Autodesk Fusion 360 part; units mm, degrees
sketch "Sketch1" plane through (0, 0, 0) normal (0, 1, 0) x (1, 0, 0)
  line L0 (-10, -10) -> (10, -10)
  line L1 (10, -10) -> (10, 10)
  line L2 (10, 10) -> (-10, 10)
  line L3 (-10, 10) -> (-10, -10)
  line L4 (0, 15) -> (15, 15)
  line L5 (15, -15) -> (-15, -15)
  line L6 (0, 15) -> (-15, 15)
  line L7 (0, -15) -> (15, -15)
  line L8 (0, -15) -> (-15, -15)
  line L9 (-15, 15) -> (15, 15)
  line L10 (-40, -12) -> (-18, -12)
  line L11 (-40, 12) -> (-18, 12)
  line L12 (40, 12) -> (18, 12)
  line L13 (40, -12) -> (18, -12)
  arc A0 (-40, 12) -> (-40, -12) centre (-40, 0) ccw
  line L14 (15, 15) -> (15, 15)
  line L15 (15, -15) -> (15, -15)
  arc A1 (40, -12) -> (40, 12) centre (40, 0) ccw
  line L16 (-15, -15) -> (-15, -15)
  line L17 (-15, 15) -> (-15, 15)
  circle A2 centre (-40, 0) radius 5
  circle A3 centre (40, 0) radius 5
  arc A4 (-18, 12) -> (-15, 15) centre (-18, 15) ccw
  arc A5 (15, 15) -> (18, 12) centre (18, 15) ccw
  arc A6 (18, -12) -> (15, -15) centre (18, -15) ccw
  arc A7 (-15, -15) -> (-18, -12) centre (-18, -15) ccw
  line L18 (-15, -15) -> (-15, 15)
  line L19 (15, 15) -> (15, -15)
  line L20 (52, 0) -> (52, 70) construction
  line L21 (-52, 0) -> (-52, 70) construction
  line L22 (0, 70) -> (-24.5, 70)
  line L23 (0, 70) -> (24.5, 70)
  line L24 (-15, 15) -> (-24.5, 70)
  line L25 (15, 15) -> (24.5, 70)
  dimension "d2" = 15
  dimension "d4" = 30
  dimension "d12" = 3
  dimension "d13" = 3
  dimension "d14" = 3
  dimension "d15" = 3
  dimension "d17" = 70
  dimension "d19" = 70
  dimension "d20" = 24.5
  dimension "d21" = 24.5
extrude "Extrude1" add sketch "Sketch1" along normal blind 15 and the other way blind 15 contours L4 L5 L6 L7 L8 L9 L18 L19
extrude "Extrude3" add sketch "Sketch1" along normal blind 5 contours L10 L11 A0 A4 A7 L18
extrude "Extrude4" add sketch "Sketch1" along normal blind 0 and the other way blind 5 contours L10 L11 A0 A4 A7 L18
extrude "Extrude5" add sketch "Sketch1" along normal blind 5 and the other way blind 5 contours L12 L13 A1 A5 A6 L19
extrude "Extrude6" add sketch "Sketch1" along normal blind 15 and the other way blind 7.5 contours L4 L6 L9 L22 L23 L24 L25
sketch "Sketch2" plane through (0, 0, 0) normal (1, 0, 0) x (0, 1, 0)
  line L0 (0, -15) -> (-7.5, -15)
  line L1 (-7.5, -15) -> (-7.5, -70)
  line L2 (-7.5, -70) -> (-30, -70)
  line L3 (-7.5, -15) -> (-30, -70)
  dimension "d44" = 7.5
  dimension "d45" = 22.5
extrude "Extrude7" add sketch "Sketch2" along normal blind 7.5 and the other way blind 7.5
sketch "Sketch3" plane through (0, 0, -70) normal (0, 0, -1) x (1, 0, 0)
  line L0 (-24.5, 7.5) -> (-24.5, -15)
  line L1 (-24.5, -15) -> (24.5, -15)
  line L2 (24.5, -15) -> (24.5, 7.5)
  line L3 (24.5, 7.5) -> (7.5, 7.5)
  line L4 (7.5, 7.5) -> (7.5, 30)
  line L5 (7.5, 30) -> (-7.5, 30)
  line L6 (-7.5, 30) -> (-7.5, 7.5)
  line L7 (-7.5, 7.5) -> (-24.5, 7.5)
  line L8 (0, -15) -> (45, -15)
  line L9 (45, -15) -> (-45, -15)
  line L10 (-45, 30) -> (45, 30)
  arc A0 (-45, -2.5) -> (-45, 17.5) centre (-45, 7.5) ccw
  arc A1 (-45, 17.5) -> (-45, -2.5) centre (-45, 7.5) ccw
  arc A2 (45, -2.5) -> (45, 17.5) centre (45, 7.5) ccw
  arc A3 (45, 17.5) -> (45, -2.5) centre (45, 7.5) ccw
  arc A4 (45, -15) -> (45, 30) centre (45, 7.5) ccw
  arc A5 (-45, 30) -> (-45, -15) centre (-45, 7.5) ccw
  line L11 (-24.5, -15) -> (24.5, -15)
  dimension "d51" = 22.5
  dimension "d52" = 20
  dimension "d53" = 20
extrude "Extrude8" add sketch "Sketch3" along normal blind 15
extrude "Extrude2" [suppressed]
The model under review builds one solid part; all positions refer to its coordinate system, in mm. A direction names the side the tool comes from. Round coordinates to 2 decimals unless told otherwise and drop trailing zeros. Order: outer loops, then holes, each group sorted by start corner. A loop starts at its lowest first (then second) coordinate and runs counter-clockwise, first axis right, second up. Notation, with made-up numbers: M 6.5,30.25 L 48.5,30.25 A16 ccw 48.5,49.25 Z; hole C -14,44.25 d5. An arc over 180 degrees is marked long. Use a Markdown table: item, result.
1) Consider section D-D (x = 42). Write out the cut boundary in (y, z).
Report:
| item | result |
|---|---|
| outline | M -30,-85 L -17.04,-85 L -17.04,-70 L -30,-70 Z; M -5,-11.83 L 5,-11.83 L 5,-4.58 L -5,-4.58 Z; M -5,4.58 L 5,4.58 L 5,11.83 L -5,11.83 Z; M 2.04,-85 L 15,-85 L 15,-70 L 2.04,-70 Z |
2) Consider section A-A (x = 5). Write out the cut boundary in (y, z), then the cut area to 3 significant figures.
Report:
| item | result |
|---|---|
| outline | M -30,-85 L 15,-85 L 15,-10 L -15,-10 L -15,-15 L -7.5,-15 L -30,-70 Z; M -15,10 L 15,10 L 15,15 L -15,15 Z |
| area | 2,830 mm^2 |
3) Wall thickness on line 1 along X through (y, z) = (0.5, 0); line 2 along X through (y, z) = (-7.5, -81); line 3 along Z through (x, y) = (-40, -1): over which ranges is each line inside the solid? List them lowest first. Write a range as [from, to].
Report:
| item | result |
|---|---|
| line 1 | [-52, -45], [-35, -10], [10, 35], [45, 52] |
| line 2 | [-67.5, -55], [-35, 35], [55, 67.5] |
| line 3 | [-12, -5], [5, 12] |
4) Tool access review of faces 1 (the face through (-34, 5, 0)), 2 (the face through (0, -11, -15)), 3 (the face through (-29, 0, -12)), 4 (the face through (-10.2, -15, -0.2)): name each direction out of +Z, -Z, +X, -X, +Y, -Y from which nothing blocks a thin tool from reaching the whole face with its end or side.
Report:
| item | result |
|---|---|
| face 1 | +Z, -X, +Y |
| face 2 | +X, -X, -Y |
| face 3 | -X, +Y, -Y |
| face 4 | +Z, +X, -X, -Y |
5) Insertion check: pin 1 (16 mm diameter, centred on y = 6.5, z = 2, fed in from +X); pin 2 (3 mm diameter, centred on y = 11, z = -6, fed in from -X); pin 3 (11 mm diameter, centred on y = -8.5, z = 7, fed in from +X). Each pin has a flat end and moves straight along its axis. Give the tip position at first contact, or say it passes through.
Report:
| item | result |
|---|---|
| pin 1 | x = 52 |
| pin 2 | x = -15 |
| pin 3 | x = 51.68 |
6) Consider section C-C (y = -3). Give the number of separate pieces and of enclosed holes in the cut face, then the cut area to 3 significant figures.
Report:
| item | result |
|---|---|
| separate pieces | 3 |
| enclosed holes | 3 |
| area | 5,650 mm^2 |
7) Draft analysis for pull direction Z (two halves, no side actions). For faces 5 (the face through (15, 10, 0)), 6 (the face through (-14, -7.5, -49)), 7 (the face through (-1, -8, -85)), state which applies: released by +Z, released by -Z, zero draft, split by the parting line, or undercut.
Report:
| item | result |
|---|---|
| face 5 | zero draft |
| face 6 | undercut |
| face 7 | released by -Z |
8) Consider section B-B (z = 0). Write out the cut boundary in (x, y).
Report:
| item | result |
|---|---|
| outline | M -52,-5 L -45,-5 L -45,5 L -52,5 Z; M -35,-5 L -15,-5 L -15,-15 L -10,-15 L -10,15 L -15,15 L -15,5 L -35,5 Z; M 10,-15 L 15,-15 L 15,-5 L 35,-5 L 35,5 L 15,5 L 15,15 L 10,15 Z; M 45,-5 L 52,-5 L 52,5 L 45,5 Z |
